The listing builds one solid part. Answer for the finished solid, in the listing's coordinates (mm). Face numbers are marked on the shaded views. Round coordinates to 2 decimals unless told otherwise and drop trailing zeros. Order: outer loops, then holes, each group sorted by start corner. A loop starts at its lowest first (then second) coordinate and runs counter-clockwise, first axis right, second up. Notation, with made-up numbers: (45.25, -15.75) - (65.25, -15.75) arc R8 ccw to (65.25, -9.75) - close; hole circle Ø1 at (-12, -3.5). An arc over 180 degrees is marked (long way). Write item = value, one per line.
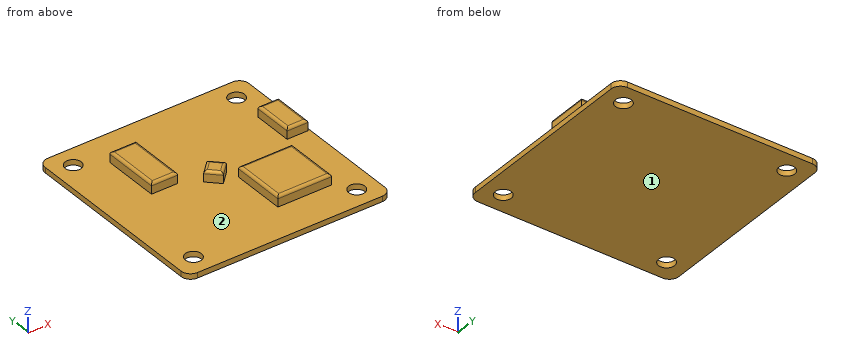
from build123d import *

# Parameters (mm, degrees)
SKETCH_R      = 1.5
PAD_DEPTH     = 1
SKETCH001_W   = 10
SKETCH001_H   = 10
SKETCH001_W_2 = 4.88679
SKETCH001_H_2 = 10.561771
SKETCH001_W_3 = 3.86214
SKETCH001_H_3 = 7.409003
PAD001_DEPTH  = 2
FILLET_R      = 0.5


with BuildPart() as part:
    # Sketch → Pad (new body)
    with BuildSketch(Plane.XY):
        with BuildLine():
            Line((-17.25, 19), (17.25, 19))
            ThreePointArc((19, 17.25), (18.487437, 18.487437), (17.25, 19))
            Line((19, 17.25), (19, -17.25))
            ThreePointArc((17.25, -19), (18.487437, -18.487437), (19, -17.25))
            Line((17.25, -19), (-17.25, -19))
            ThreePointArc((-19, -17.25), (-18.487437, -18.487437), (-17.25, -19))
            Line((-19, -17.25), (-19, 17.25))
            ThreePointArc((-17.25, 19), (-18.487437, 18.487437), (-19, 17.25))
        make_face()
        with Locations((15.25, 15.25)):
            Circle(SKETCH_R, mode=Mode.SUBTRACT)
        with Locations((-15.25, -15.25)):
            Circle(SKETCH_R, mode=Mode.SUBTRACT)
        with Locations((-15.25, 15.25)):
            Circle(SKETCH_R, mode=Mode.SUBTRACT)
        with Locations((15.25, -15.25)):
            Circle(SKETCH_R, mode=Mode.SUBTRACT)
    extrude(amount=PAD_DEPTH)

    # Sketch001 (on Face14 of Pad) → Pad001 (join)
    with BuildSketch(Plane.XY.offset(1)):
        with Locations((7.881429, -7.044085)):
            Rectangle(SKETCH001_W, SKETCH001_H)
        Polygon((0, -2.12132), (2.12132, 0), (0, 2.12132), (-2.12132, 0), align=None)
        with Locations((-7.939527, 7.278862)):
            Rectangle(SKETCH001_W_2, SKETCH001_H_2)
        with Locations((16.691468, 5.466022)):
            Rectangle(SKETCH001_W_3, SKETCH001_H_3)
    extrude(amount=PAD001_DEPTH)

    # Fillet
    fillet_edges = [part.edges().sort_by_distance(p)[0] for p in [
        (1.06066, -1.06066, 3),
        (1.06066, 1.06066, 3),
        (-1.06066, 1.06066, 3),
        (-1.06066, -1.06066, 3),
        (7.881429, -2.044085, 3),
        (12.881429, -7.044085, 3),
        (7.881429, -12.044085, 3),
        (2.881429, -7.044085, 3),
        (-7.939527, 12.559748, 3),
        (-5.496132, 7.278863, 3),
        (-7.939527, 1.997977, 3),
        (-10.382922, 7.278863, 3),
        (16.691468, 9.170523, 3),
        (18.622538, 5.466022, 3),
        (16.691468, 1.76152, 3),
        (14.760398, 5.466022, 3),
    ]]
    fillet(fillet_edges, radius=FILLET_R)


solid = part.part
Q1. Section D-D on x = 6.5 is taken. Determine the outline of the cut face in (y, z).
Model answer:
outline = (-19, 0) - (19, 0) - (19, 1) - (-2.04, 1) - (-2.04, 2.5) arc R0.5 ccw to (-2.54, 3) - (-11.54, 3) arc R0.5 ccw to (-12.04, 2.5) - (-12.04, 1) - (-19, 1) - close
Q2. Find the intervals of material crossed by line 1 (Y direction, x = 15.25, z = 0.7); line 2 (X direction, y = -15, z = 0.7); line 3 (Z direction, x = 14, y = -13), in increasing order. Write a range as from..to.
Model answer:
line_1 = -19..-16.75, -13.75..13.75, 16.75..19
line_2 = -19..-16.73, -13.77..13.77, 16.73..19
line_3 = 0..1
Q3. Flat-ended cylindrical pins translate along their axes: P1, Ø0.8, axis at x = 16.5, z = 1.5, coming from the -Y side; P2, Ø0.8, axis at x = 5.5, z = 1.5, coming from the +Y side; P3, Ø0.8, axis at x = 16.5, z = 2, coming from the +Y side. Find the tip coordinate at first contact, or state that the pin passes through.
Model answer:
P1 = 1.76
P2 = -2.04
P3 = 9.17
Q4. Section A-A on y = -15.25 is taken. Determine the outline of the cut face in (x, z).
Model answer:
outline = (-19, 0) - (-16.75, 0) - (-16.75, 1) - (-19, 1) - close; (-13.75, 0) - (13.75, 0) - (13.75, 1) - (-13.75, 1) - close; (16.75, 0) - (19, 0) - (19, 1) - (16.75, 1) - close
Q5. Determine the mould class of the marked faces 1 and 2 for opening direction X: released by +X, released by -X, zero draft, split by the parting line, or undercut.
Model answer:
face_1 = zero draft
face_2 = undercut
Q6. Section C-C on z = 0.5 is taken. Determine the outline of the cut face in (x, y).
Model answer:
outline = (-19, -17.25) arc R1.75 ccw to (-17.25, -19) - (17.25, -19) arc R1.75 ccw to (19, -17.25) - (19, 17.25) arc R1.75 ccw to (17.25, 19) - (-17.25, 19) arc R1.75 ccw to (-19, 17.25) - close; hole circle Ø3 at (-15.25, -15.25); hole circle Ø3 at (-15.25, 15.25); hole circle Ø3 at (15.25, -15.25); hole circle Ø3 at (15.25, 15.25)
